Source: three-view drawing plus pictorial views. Frame: mm from the lowest corner of the part. A direction names the side the tool comes from. Coordinates: 2 decimals unless noted, no trailing zeros. Loops run counter-clockwise (first coordinate to the right, second up) from the corner with the lowest first, then second, coordinate; pieces in that order, holes last.
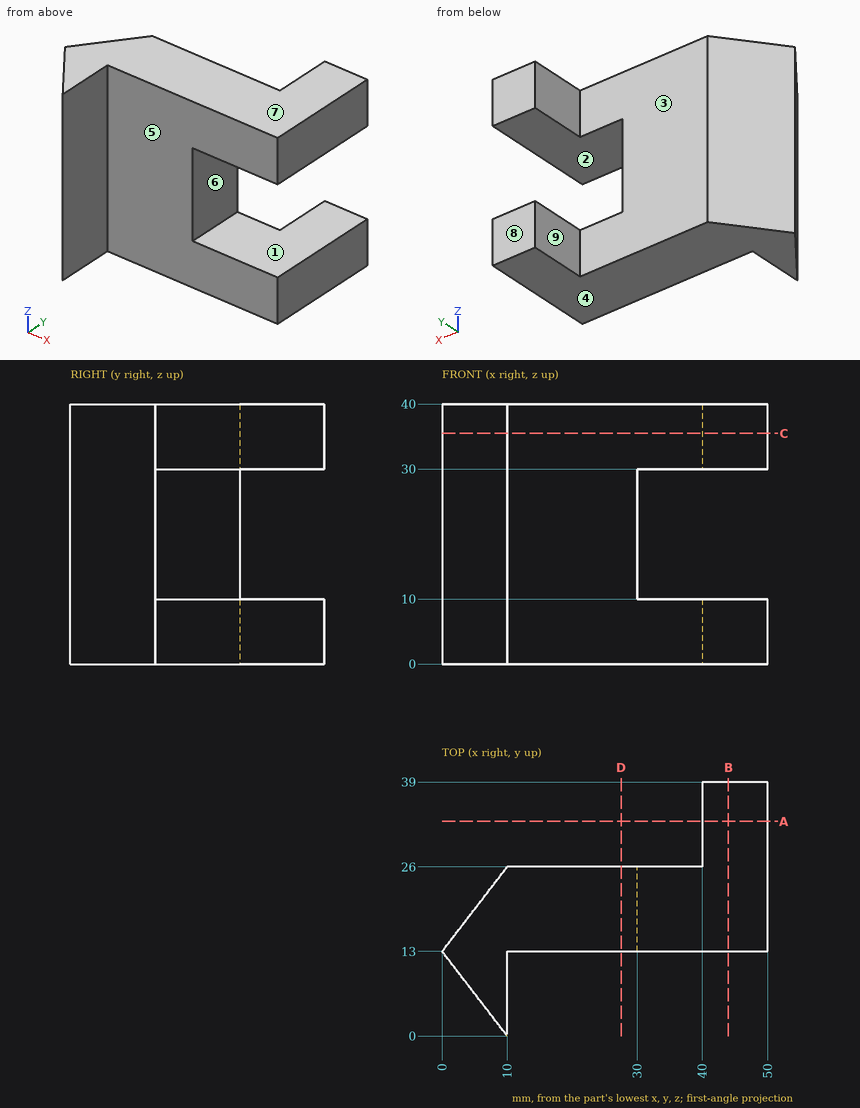
Q1. Section D-D, the plane x = 27.5. Return the cut outline in (y, z), plus the area to 3 significant figures.
Q2. Line query: line 1 along Z through (x, y) = (41, 32); line 2 along Y through (x, z) = (15, 28); line 3 along Y through (x, z) = (45, 2). Output: solid intervals per line, ascending.
Q3. Contact query for flat-ended pins moving along their axis: pin 1 Ø6.5 at (y, z) = (3.5, 21) entering from +X; pin 2 Ø6.5 at (y, z) = (19, 17) entering from +X; pin 3 Ø2 at (y, z) = (8, 9.5) entering from -X. Output: stop coordinate, or through.
Q4. Draft query along Z for the marked faces 1, 2, 3 and 4. Return one class per face: +Z half, -Z half, draft (parallel to the pull), parting line (faces both ways), or undercut.
Q5. Section C-C, the plane z = 35.5. Return the cut outline in (x, y), plus the area to 3 significant figures.
Q6. Section A-A, the plane y = 33. Return the cut outline in (x, z), plus the area to 3 significant figures.
Q7. Section B-B, the plane x = 44. Return the cut outline in (y, z).
Q8. Access query for the marked faces 5, 6, 7, 8 and 9. Directions: +Z, -Z, +X, -X, +Y, -Y. A direction counts if a zero-diameter tool reaches every point of the face in a straight line with its end or side. Return the directions, or none.
Derived:
1. outline: (13, 0) - (26, 0) - (26, 40) - (13, 40) - close
1. area: 520 mm2
2. line 1: z = 0 to 10, 30 to 40
2. line 2: y = 13 to 26
2. line 3: y = 13 to 39
3. pin 1: stops at x = 10
3. pin 2: stops at x = 30
3. pin 3: stops at x = 3.08
4. face 1: undercut
4. face 2: undercut
4. face 3: draft
4. face 4: -Z half
5. outline: (0, 13) - (10, 0) - (10, 13) - (50, 13) - (50, 39) - (40, 39) - (40, 26) - (10, 26) - close
5. area: 780 mm2
6. outline: (40, 0) - (50, 0) - (50, 10) - (40, 10) - close; (40, 30) - (50, 30) - (50, 40) - (40, 40) - close
6. area: 200 mm2
7. outline: (13, 0) - (39, 0) - (39, 10) - (13, 10) - close; (13, 30) - (39, 30) - (39, 40) - (13, 40) - close
8. face 5: +Z, -Z, +X, -Y
8. face 6: +X, +Y, -Y
8. face 7: +Z, +X, -X, +Y, -Y
8. face 8: +Z, -Z, +X, -X, +Y
8. face 9: +Z, -Z, -X, +Y
